from build123d import *

# Parameters (mm, degrees)
BOSS_EXTRUDE1_DEPTH = 430
CHAMFER1_SIZE       = 0.5
LPATTERN1_COUNT     = 11
LPATTERN1_PITCH     = 40


with BuildPart() as part:
    # Sketch1 → Boss-Extrude1 (new body)
    with BuildSketch(Plane.XY):
        with BuildLine():
            Line((-7.5, 10), (7.5, 10))
            Line((7.5, 10), (7.5, 8.25))
            Line((7.5, 8.25), (7.5, 8.030776406))
            ThreePointArc((7.5, 8.030776406), (6.865647614, 7.812463569), (6.5, 7.25))
            Line((6.5, 7.25), (6, 7.25))
            Line((6, 7.25), (6, 6.75))
            Line((6, 6.75), (6.5, 6.75))
            ThreePointArc((6.5, 6.75), (6.865647614, 6.187536431), (7.5, 5.969223594))
            Line((7.5, 5.969223594), (7.5, 5.75))
            Line((7.5, 5.75), (7.5, 0))
            Line((7.5, 0), (-7.5, 0))
            Line((-7.5, 0), (-7.5, 5.75))
            Line((-7.5, 5.75), (-7.5, 5.969223594))
            ThreePointArc((-7.5, 5.969223594), (-6.865647614, 6.187536431), (-6.5, 6.75))
            Line((-6.5, 6.75), (-6, 6.75))
            Line((-6, 6.75), (-6, 7.25))
            Line((-6, 7.25), (-6.5, 7.25))
            ThreePointArc((-6.5, 7.25), (-6.865647614, 7.812463569), (-7.5, 8.030776406))
            Line((-7.5, 8.030776406), (-7.5, 8.25))
            Line((-7.5, 8.25), (-7.5, 10))
        make_face()
    extrude(amount=BOSS_EXTRUDE1_DEPTH)

    # Chamfer1
    chamfer1_edges = [part.edges().sort_by_distance(p)[0] for p in [
        (-7.5, 10, 215),
        (7.5, 10, 215),
        (7.5, 0, 215),
        (-7.5, 0, 215),
    ]]
    chamfer(chamfer1_edges, length=CHAMFER1_SIZE)

    # Sketch3 → M3 六角承窩頭蓋螺釘的柱孔1 (revolve, cut)
    with BuildSketch(Plane(origin=(0, 10, 15), x_dir=(0, 0, 1), z_dir=(1, 0, 0))):
        Polygon((0, 0), (0, 10), (2, 10), (1.75, 9.75), (1.75, 4.5), (3, 4.5), (3, 0.5), (3.5, 0), align=None)
    hole_wizard_m3_1 = revolve(axis=Axis((0, 16.35, 15), (0, -1, 0)), mode=Mode.SUBTRACT)

    # LPattern1: M3 六角承窩頭蓋螺釘的柱孔1 ×11
    with Locations(*[(0, 0, i * LPATTERN1_PITCH) for i in range(1, LPATTERN1_COUNT)]):
        add(hole_wizard_m3_1, mode=Mode.SUBTRACT)


solid = part.part
Model file for the job. Use its own axes, mm. Give positions to 0.01 mm unless a question says otherwise; leave off trailing zeros. Write each loop counter-clockwise with the first axis right and the second up, starting at its lowest first coordinate (ties: lowest second). Pieces come first, ordered by that corner, then holes. Notation, with made-up numbers: M -35,47.5 L -14,47.5 A9 cw -14,54.5 Z; hole C 8.5,35.25 d3. An arc over 180 degrees is marked long. One line per item, written item: value. Start each with the question number.
Q1. Saw through at B-B, the plane z = 205. Write the cut outline in (x, y).
Q2. Probe probe 1 along X at (y, z) = (1.35, 135); probe 2 along X at (y, z) = (7.15, 255); probe 3 along X at (y, z) = (6.5, 26). List the from-to ranges inside material, lowest first. Write a range as [from, to].
Q3. Drop flat-ended pins along their axis: pin 1 Ø6 at (y, z) = (6, 252) entering from +X; pin 2 Ø0.6 at (y, z) = (7, 204.5) entering from -X; pin 3 Ø5 at (x, z) = (0.5, 55.5) entering from +Y; pin 4 Ø5 at (x, z) = (0, 135) entering from +Y. Give the stop position or say it passes through.
Q4. Saw through at A-A, the plane y = 3.5. State how many separate pieces and enclosed holes the cut face has, plus the area to 3 significant figures.
Output values:
1. outline: M -7.5,0.5 L -7,0 L 7,0 L 7.5,0.5 L 7.5,5.97 A1.03 cw 6.5,6.75 L 6,6.75 L 6,7.25 L 6.5,7.25 A1.03 cw 7.5,8.03 L 7.5,9.5 L 7,10 L -7,10 L -7.5,9.5 L -7.5,8.03 A1.03 cw -6.5,7.25 L -6,7.25 L -6,6.75 L -6.5,6.75 A1.03 cw -7.5,5.97 Z
2. probe 1: x = [-7.5, -1.75], [1.75, 7.5]
2. probe 2: x = [-6, -3], [3, 6]
2. probe 3: x = [-6.6, 6.6]
3. pin 1: stops at x = 7.5
3. pin 2: stops at x = -6.51
3. pin 3: stops at y = 9.71
3. pin 4: stops at y = 5.5
4. separate pieces: 1
4. enclosed holes: 11
4. area: 6,340 mm²
